For this review, take the finished solid that the model builds, in its own axes (mm). A direction names the side the tool comes from. Give positions to 0.01 mm unless a question says otherwise; leave off trailing zeros. Write each loop counter-clockwise with the first axis right and the second up, starting at its lowest first coordinate (ties: lowest second). Pieces come first, ordered by that corner, then holes. Notation, with made-up numbers: M 50.25,18 L 99.25,18 A29 ccw 99.25,42 Z; hole C -29,47 d8. An arc over 180 degrees is marked long. Answer as a JSON object with one key per item and string values. Group by question number.
```python
from build123d import *

# Parameters (mm, degrees)
F0_W     = 102
F0_H     = 40
F1_DEPTH = 3
F2_W     = 3
F2_H     = 5
F3_DEPTH = 3
F4_W     = 5
F4_H     = 3
F5_DEPTH = 3
F6_W     = 109.860795
F6_H     = 22.121532
F7_DEPTH = 25


with BuildPart() as f1:
    # F0 (on Front) → F1 (new body)
    with BuildSketch(Plane.XZ):
        Rectangle(F0_W, F0_H)
    extrude(amount=F1_DEPTH)

    # F2 (on face) → F3 (join)
    with BuildSketch(Plane.XZ.offset(3)):
        with Locations((-52.5, -17.5)):
            Rectangle(F2_W, F2_H)
        with Locations((-52.5, -7.5)):
            Rectangle(F2_W, F2_H)
        with Locations((-52.5, 2.5)):
            Rectangle(F2_W, F2_H)
        with Locations((-52.5, 12.5)):
            Rectangle(F2_W, F2_H)
        with Locations((52.5, -7.5)):
            Rectangle(F2_W, F2_H)
        with Locations((52.5, -17.5)):
            Rectangle(F2_W, F2_H)
        with Locations((52.5, 12.5)):
            Rectangle(F2_W, F2_H)
        with Locations((52.5, 2.5)):
            Rectangle(F2_W, F2_H)
    extrude(amount=-F3_DEPTH)

    # F4 (on face) → F5 (join)
    with BuildSketch(Plane.XZ.offset(3)):
        with Locations((5, -21.5)):
            Rectangle(F4_W, F4_H)
        with Locations((15, -21.5)):
            Rectangle(F4_W, F4_H)
        with Locations((25, -21.5)):
            Rectangle(F4_W, F4_H)
        with Locations((35, -21.5)):
            Rectangle(F4_W, F4_H)
        with Locations((45, -21.5)):
            Rectangle(F4_W, F4_H)
        with Locations((-25, -21.5)):
            Rectangle(F4_W, F4_H)
        with Locations((-15, -21.5)):
            Rectangle(F4_W, F4_H)
        with Locations((-5, -21.5)):
            Rectangle(F4_W, F4_H)
        with Locations((-35, -21.5)):
            Rectangle(F4_W, F4_H)
        with Locations((-45, -21.5)):
            Rectangle(F4_W, F4_H)
    extrude(amount=-F5_DEPTH)

    # F6 (on face) → F7 (cut)
    with BuildSketch(Plane.XZ.offset(3)):
        with Locations((0.930397, 11.060766)):
            Rectangle(F6_W, F6_H)
    extrude(amount=-F7_DEPTH, mode=Mode.SUBTRACT)


solid = f1.part
```
Item 1: Consider section A-A (x = 1). Give the boundary of the cut face in (y, z), plus the area to 3 significant figures.
Item 2: Draft analysis for pull direction X (two halves, no side actions). For faces 4 (the flat face through (-25, -2, -23)), 5 (the flat face through (17.5, -2, -22)), 6 (the flat face through (-54, -2, -8)), state which applies: released by +X, released by -X, zero draft, split by the parting line, or undercut.
Item 3: Consider section B-B (z = -3.5). Give the boundary of the cut face in (x, y), plus the area to 3 significant figures.
Item 4: Machinability: for faces 1 (the flat face through (-51, -1, -3)), 2 (the flat face through (51, -1, -13)), 3 (the flat face through (-32.5, -2, -22)), which of the approach directions +Z, -Z, +X, -X, +Y, -Y give a long, thin tool a straight path to every point of the face, cutting with its end or side? Answer none if there is none.
Item 5: Insertion check: P1, Ø1.5, axis at y = -1.5, z = -21.5, coming from the -X side; P2, Ø1.5, axis at y = -1, z = -3.5, coming from the -X side; P3, Ø1.5, axis at y = -1, z = -22, coming from the +X side. Each pin has a flat end and moves straight along its axis. Give the tip position at first contact, or say it passes through.
Item 6: To check wall thickness, follow probe 1 along Z at (x, y) = (18.5, -1.8); probe 2 along X at (y, z) = (-2.5, -11.5). State the ranges of each line that lie inside material, in increasing order.
Result set:
{
 "1": {"outline": "M -3,-20 L 0,-20 L 0,0 L -3,0 Z", "area": "60.0 mm^2"},
 "2": {"face 4": "zero draft", "face 5": "undercut", "face 6": "released by -X"},
 "3": {"outline": "M -51,-3 L 51,-3 L 51,0 L -51,0 Z", "area": "306 mm^2"},
 "4": {"face 1": "+Z, -X, +Y, -Y", "face 2": "+X, +Y, -Y", "face 3": "-Z, +Y, -Y"},
 "5": {"P1": "stops at x = -47.5", "P2": "stops at x = -51", "P3": "stops at x = 47.5"},
 "6": {"probe 1": "z = -20 to 0", "probe 2": "x = -51 to 51"}
}
